Can you work these out from the model? Positions are in its coordinate system, mm. Face numbers are marked on the shaded views. A direction names the side the tool comes from. Round coordinates to 2 decimals unless told otherwise and drop trailing zeros. Write each loop counter-clockwise with the first axis right and the second up, starting at its lowest first coordinate (ties: lowest second). Pieces come first, ordered by that corner, then holes. Notation, with made-up numbers: M 27,29 L 45,29 A15 cw 45,56 Z; hole C 53,73 d7. An arc over 180 degrees is marked long. Use one line per item in the form item = value. Start each with the question number.
```python
from build123d import *

# Parameters (mm, degrees)
ESQUISSE1_R      = 13
EXTRUSION1_DEPTH = 1
ESQUISSE2_R      = 10.875
EXTRUSION2_DEPTH = 8
ESQUISSE3_R      = 13
EXTRUSION3_DEPTH = 1
ESQUISSE4_R      = 8
EXTRUSION4_DEPTH = 6
ESQUISSE5_R      = 2
EXTRUSION5_DEPTH = 25.372115214


with BuildPart() as part:
    # Esquisse1 → Extrusion1 (new body)
    with BuildSketch(Plane(origin=(0, 0, 0), x_dir=(1, 0, 0), z_dir=(0, 1, 0))):
        with Locations(Location((0, 0, 0), (0, 0, 270))):
            Circle(ESQUISSE1_R)
    extrude(amount=EXTRUSION1_DEPTH)

    # Esquisse2 → Extrusion2 (add)
    with BuildSketch(Plane(origin=(0, 1, 0), x_dir=(-1, 0, 0), z_dir=(0, 1, 0))):
        with Locations(Location((0, 0, 0), (0, 0, 90))):
            Circle(ESQUISSE2_R)
    extrude(amount=EXTRUSION2_DEPTH)

    # Esquisse3 → Extrusion3 (add)
    with BuildSketch(Plane(origin=(0, 9, 0), x_dir=(-1, 0, 0), z_dir=(0, 1, 0))):
        with Locations(Location((0, 0, 0), (0, 0, 90))):
            Circle(ESQUISSE3_R)
    extrude(amount=EXTRUSION3_DEPTH)

    # Esquisse4 → Extrusion4 (add)
    with BuildSketch(Plane(origin=(0, 10, 0), x_dir=(-1, 0, 0), z_dir=(0, 1, 0))):
        with Locations(Location((0, 0, 0), (0, 0, 90))):
            Circle(ESQUISSE4_R)
    extrude(amount=EXTRUSION4_DEPTH)

    # Esquisse5 → Extrusion5 (cut, through all)
    with BuildSketch(Plane(origin=(0, 16, 0), x_dir=(-1, 0, 0), z_dir=(0, 1, 0))):
        with Locations(Location((0, 0, 0), (0, 0, 90))):
            Circle(ESQUISSE5_R)
    extrude(amount=-EXTRUSION5_DEPTH, mode=Mode.SUBTRACT)


solid = part.part
```
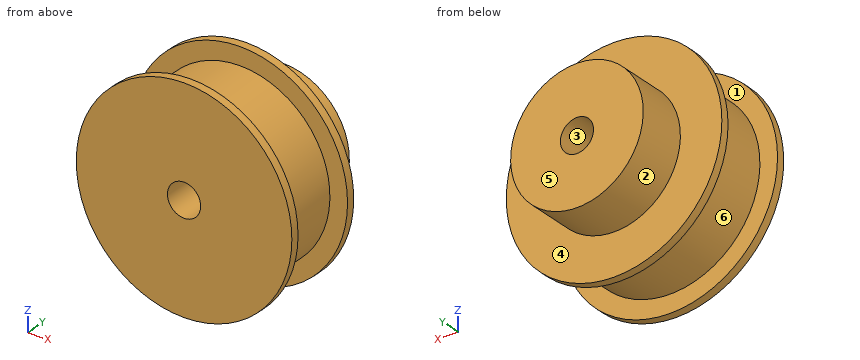
1. If we section it at D-D (x = 6.75): List the corners of the cut face in (y, z) for me.
2. Which directions (+Z, -Z, +X, -X, +Y, -Y) give clear straight access to the entire face, cutting with the end or side of a thin tool? Please do the marked faces 4, 5 and 6.
3. If we section it at A-A (x = 0): List the corners of the cut face in (y, z) for me (3 decimals).
4. If we section it at B-B (z = 0): List the corners of the cut face in (x, y) for me (3 decimals).
5. If we section it at C-C (y = 12): List the corners of the cut face in (x, z) for me, and give its area (3 significant figures).
6. Please list where these lines run through material, in increasing order: line 1 along Y through (x, z) = (-10, -6); line 2 along Y through (x, z) = (3, -9.25); line 3 along X through (y, z) = (10.75, -1.25).
7. If we mould it in two halves opening along X, with no side actions, what happens to the marked faces 1, 2 and 3? For each: pulls with the +X half, pulls with the -X half, needs draft (parallel to the pull), parting line crosses it, or undercut.
8. Will these pins go through, and if not, where does the flat tip stop? pin 1 (5 mm diameter, centred on y = 13, z = -6, fed in from -X); pin 2 (4 mm diameter, centred on y = 8.5, z = 8, fed in from -X); pin 3 (1 mm diameter, centred on y = 10, z = -5.5, fed in from +X).
Model answer:
q1.outline = M 0,-11.11 L 1,-11.11 L 1,-8.53 L 9,-8.53 L 9,-11.11 L 10,-11.11 L 10,-4.29 L 16,-4.29 L 16,4.29 L 10,4.29 L 10,11.11 L 9,11.11 L 9,8.53 L 1,8.53 L 1,11.11 L 0,11.11 Z
q2.face_4 = +Y
q2.face_5 = +Z, -Z, +X, -X, +Y
q2.face_6 = none
q3.outline = M 0,-13 L 1,-13 L 1,-10.875 L 9,-10.875 L 9,-13 L 10,-13 L 10,-8 L 16,-8 L 16,-2 L 0,-2 Z; M 0,2 L 16,2 L 16,8 L 10,8 L 10,13 L 9,13 L 9,10.875 L 1,10.875 L 1,13 L 0,13 Z
q4.outline = M -13,0 L -2,0 L -2,16 L -8,16 L -8,10 L -13,10 L -13,9 L -10.875,9 L -10.875,1 L -13,1 Z; M 2,0 L 13,0 L 13,1 L 10.875,1 L 10.875,9 L 13,9 L 13,10 L 8,10 L 8,16 L 2,16 Z
q5.outline = C 0,0 d16; hole C 0,0 d4
q5.area = 188 mm2
q6.line_1 = 0 to 1, 9 to 10
q6.line_2 = 0 to 10
q6.line_3 = -7.9 to -1.56, 1.56 to 7.9
q7.face_1 = needs draft
q7.face_2 = parting line crosses it
q7.face_3 = undercut
q8.pin_1 = -7.19
q8.pin_2 = -11.5
q8.pin_3 = 12
